from build123d import *

# Parameters (mm, degrees)
SKETCH1_R           = 8.3
BOSS_EXTRUDE1_DEPTH = 80.34
SKETCH2_R           = 1.4
BOSS_EXTRUDE2_DEPTH = 0.5
DOME1_FACE_RADIUS   = 1.4
DOME1_HEIGHT        = 1.4
SKETCH3_R           = 4.4
BOSS_EXTRUDE3_DEPTH = 12.5
BOSS_EXTRUDE3_TAPER = 3.2
SKETCH4_R           = 4.45
BOSS_EXTRUDE4_DEPTH = 1.5
SKETCH5_R           = 4.45
BOSS_EXTRUDE5_DEPTH = 3.32
BOSS_EXTRUDE5_TAPER = 8.5
SKETCH6_R           = 2.85
BOSS_EXTRUDE6_DEPTH = 10


with BuildPart() as part:
    # Sketch1 → Boss-Extrude1 (new body)
    with BuildSketch(Plane.XY):
        Circle(SKETCH1_R)
    extrude(amount=BOSS_EXTRUDE1_DEPTH)

    # Sketch2 → Boss-Extrude2 (add)
    with BuildSketch(Plane.XY.offset(80.34)):
        with Locations((0, 5.73)):
            Circle(SKETCH2_R)
    extrude(amount=BOSS_EXTRUDE2_DEPTH)

    # Dome1: a dome of height H over a round flat face of radius A is a cap of a sphere of radius (A * A + H * H) / (2 * H)
    dome1_r = (DOME1_FACE_RADIUS * DOME1_FACE_RADIUS + DOME1_HEIGHT * DOME1_HEIGHT) / (2 * DOME1_HEIGHT)
    dome1_base = Plane((0, 5.73, 80.84), z_dir=(0, 0, 1))
    with Locations(dome1_base.offset(DOME1_HEIGHT - dome1_r)):
        dome1_ball = Sphere(dome1_r, mode=Mode.PRIVATE)
    add(split(dome1_ball, bisect_by=dome1_base, keep=Keep.TOP, mode=Mode.PRIVATE))

    # Sketch3 → Boss-Extrude3 (add)
    with BuildSketch(Plane.XY.offset(80.34)):
        with Locations((0, -3)):
            Circle(SKETCH3_R)
    extrude(amount=BOSS_EXTRUDE3_DEPTH, taper=BOSS_EXTRUDE3_TAPER)

    # Sketch4 → Boss-Extrude4 (add)
    with BuildSketch(Plane.XY.offset(92.84)):
        with Locations((0, -3)):
            Circle(SKETCH4_R)
    extrude(amount=BOSS_EXTRUDE4_DEPTH)

    # Sketch5 → Boss-Extrude5 (add)
    with BuildSketch(Plane.XY.offset(94.34)):
        with Locations((0, -3)):
            Circle(SKETCH5_R)
    extrude(amount=BOSS_EXTRUDE5_DEPTH, taper=BOSS_EXTRUDE5_TAPER)

    # Sketch6 → Boss-Extrude6 (add)
    with BuildSketch(Plane.XY.offset(97.66)):
        with Locations((0, -3)):
            Circle(SKETCH6_R)
    extrude(amount=BOSS_EXTRUDE6_DEPTH)


solid = part.part
Input: part model. Units: mm. Frame: model coordinates. A direction names the side the tool comes from. Coordinates: 2 decimals unless noted, no trailing zeros. Order: outer loops, then holes, each group sorted by start corner. A loop starts at its lowest first (then second) coordinate and runs counter-clockwise, first axis right, second up. Notation, with made-up numbers: M -3,24 L 15,24 A33 cw 15,59 Z; hole C -15,2.25 d9. An arc over 180 degrees is marked long. Answer in a Markdown table with one row per item.
(1) Section query A-A, the plane y = 5.73. Output: boundary loops of the cut face in (x, z).
Numbers:
| item | result |
|---|---|
| outline | M -6,0 L 6,0 L 6,80.34 L 1.4,80.34 L 1.4,80.84 A1.4 ccw -1.4,80.84 L -1.4,80.34 L -6,80.34 Z |
(2) Access query for faces 1 (the flat face through (-4, -2, 92.84)), 2 (the flat face through (0, 0, 0)), 3 (the flat face through (1, -6, 97.66)). Directions: +Z, -Z, +X, -X, +Y, -Y. A direction counts if a zero-diameter tool reaches every point of the face in a straight line with its end or side. Return the directions, or none.
Numbers:
| item | result |
|---|---|
| face 1 | none |
| face 2 | -Z, +X, -X, +Y, -Y |
| face 3 | +Z |
(3) Section query D-D, the plane y = -3. Output: boundary loops of the cut face in (x, z), plus the area to 3 significant figures.
Numbers:
| item | result |
|---|---|
| outline | M -7.74,0 L 7.74,0 L 7.74,80.34 L 4.4,80.34 L 3.7,92.84 L 4.45,92.84 L 4.45,94.34 L 3.95,97.66 L 2.85,97.66 L 2.85,107.66 L -2.85,107.66 L -2.85,97.66 L -3.95,97.66 L -4.45,94.34 L -4.45,92.84 L -3.7,92.84 L -4.4,80.34 L -7.74,80.34 Z |
| area | 1,440 mm^2 |
(4) Section query C-C, the plane x = 0. Output: boundary loops of the cut face in (y, z).
Numbers:
| item | result |
|---|---|
| outline | M -8.3,0 L 8.3,0 L 8.3,80.34 L 7.13,80.34 L 7.13,80.84 A1.4 ccw 4.33,80.84 L 4.33,80.34 L 1.4,80.34 L 0.7,92.84 L 1.45,92.84 L 1.45,94.34 L 0.95,97.66 L -0.15,97.66 L -0.15,107.66 L -5.85,107.66 L -5.85,97.66 L -6.95,97.66 L -7.45,94.34 L -7.45,92.84 L -6.7,92.84 L -7.4,80.34 L -8.3,80.34 Z |
(5) Contact query for flat-ended pins moving along their axis: pin 1 Ø1 at (y, z) = (2.5, 65) entering from +X; pin 2 Ø1 at (x, y) = (-4, -2.5) entering from +Z. Output: stop coordinate, or through.
Numbers:
| item | result |
|---|---|
| pin 1 | stops at x = 8.06 |
| pin 2 | stops at z = 97.66 |
(6) Section query B-B, the plane z = 24. Output: boundary loops of the cut face in (x, y), plus the area to 3 significant figures.
Numbers:
| item | result |
|---|---|
| outline | C 0,0 d16.6 |
| area | 216 mm^2 |
(7) Material intervals for line 1 (Z direction, x = 5.75, y = -3); line 2 (X direction, y = -0.25, z = 53); line 3 (Y direction, x = -0.25, z = 100), sorted ascending. Write a range as [from, to].
Numbers:
| item | result |
|---|---|
| line 1 | z = [0, 80.34] |
| line 2 | x = [-8.3, 8.3] |
| line 3 | y = [-5.84, -0.16] |
